```python
from build123d import *

# Parameters (mm, degrees)
F0_R     = 2.921
F1_DEPTH = 50.8
F3_DEPTH = 278.638
F4_R     = 5.08
F6_DEPTH = 79.502
F9_DEPTH = 68.072


with BuildPart() as f1:
    # F0 (on Front) → F1 (new body)
    with BuildSketch(Plane.XZ):
        Polygon((25.4, 69.85), (0, 0), (127, 0), (101.6, 69.85), align=None)
        with Locations((38.1, 53.975)):
            Circle(F0_R, mode=Mode.SUBTRACT)
        with Locations((88.9, 53.975)):
            Circle(F0_R, mode=Mode.SUBTRACT)
    extrude(amount=F1_DEPTH)

    # F2 (on Right) → F3 (cut)
    with BuildSketch(Plane.YZ):
        with BuildLine():
            Line((-38.354, 86.910382), (-38.354, 38.354))
            ThreePointArc((-38.354, 38.354), (-25.4, 25.4), (-12.446, 38.354))
            Line((-12.446, 38.354), (-12.446, 88.236041))
            Line((-12.446, 88.236041), (-38.354, 86.910382))
        make_face()
    extrude(amount=F3_DEPTH, mode=Mode.SUBTRACT)

    # F4
    f4_edges = [f1.edges().sort_by_distance(p)[0] for p in [
        (114.3, -50.8, 34.925),
        (63.5, -50.8, 69.85),
        (12.7, -50.8, 34.925),
        (101.6, -44.577, 69.85),
        (101.6, -6.223, 69.85),
        (25.4, -44.577, 69.85),
        (25.4, -6.223, 69.85),
        (63.5, 0, 69.85),
        (114.3, 0, 34.925),
        (12.7, 0, 34.925),
    ]]
    fillet(f4_edges, radius=F4_R)

    # F5 (on face) → F6 (cut)
    with BuildSketch(Plane(origin=(0, 0, 0), x_dir=(1, 0, 0), z_dir=(0, 0, -1))):
        with BuildLine():
            Line((28.321, 25.4), (31.75, 25.4))
            Line((31.75, 25.4), (35.179, 25.4))
            ThreePointArc((35.179, 25.4), (31.75, 28.829), (28.321, 25.4))
        make_face()
        with BuildLine():
            Line((35.179, 25.4), (31.75, 25.4))
            Line((31.75, 25.4), (28.321, 25.4))
            ThreePointArc((28.321, 25.4), (31.75, 21.971), (35.179, 25.4))
        make_face()
        with BuildLine():
            ThreePointArc((98.679, 25.4), (95.25, 28.829), (91.821, 25.4))
            ThreePointArc((91.821, 25.4), (95.25, 21.971), (98.679, 25.4))
        make_face()
    extrude(amount=-F6_DEPTH, mode=Mode.SUBTRACT)

    # F8 (on offset) → F9 (cut)
    with BuildSketch(Plane.XY.offset(12.7)):
        with BuildLine():
            ThreePointArc((40.64, -25.4), (31.75, -16.51), (22.86, -25.4))
            Line((22.86, -25.4), (31.75, -25.4))
            Line((31.75, -25.4), (40.64, -25.4))
        make_face()
        with BuildLine():
            ThreePointArc((104.14, -25.4), (95.25, -16.51), (86.36, -25.4))
            ThreePointArc((86.36, -25.4), (95.25, -34.29), (104.14, -25.4))
        make_face()
        with BuildLine():
            Line((31.75, -25.4), (22.86, -25.4))
            ThreePointArc((22.86, -25.4), (31.75, -34.29), (40.64, -25.4))
            Line((40.64, -25.4), (31.75, -25.4))
        make_face()
    extrude(amount=F9_DEPTH, mode=Mode.SUBTRACT)


solid = f1.part
```
Part model, mm, in its own coordinate system. A direction names the side the tool comes from. Round coordinates to 2 decimals unless told otherwise and drop trailing zeros. Loops run counter-clockwise (first coordinate to the right, second up) from the corner with the lowest first, then second, coordinate; pieces in that order, holes last.
1. Flat gauge pins, fed straight in: pin 1 (5.5 mm diameter, centred on x = 96.5, y = -25.5, fed in from +Z); pin 2 (7.5 mm diameter, centred on x = 38.1, z = 53.975, fed in from +Y); pin 3 (4.5 mm diameter, centred on x = 88.9, z = 53.975, fed in from -Y); pin 4 (4 mm diameter, centred on y = -41, z = 60, fed in from +X). Where does each tip first touch, or does it go through?
Solutions:
pin 1: stops at z = 12.7
pin 2: stops at y = 0
pin 3: passes through
pin 4: stops at x = 105.91
2. Slice it at A-A (y = -25.4). Give the cut face in (x, z).
Solutions:
outline: (0, 0) - (28.32, 0) - (28.32, 12.7) - (22.86, 12.7) - (22.86, 25.4) - (9.24, 25.4) - close; (35.18, 0) - (91.82, 0) - (91.82, 12.7) - (86.36, 12.7) - (86.36, 25.4) - (40.64, 25.4) - (40.64, 12.7) - (35.18, 12.7) - close; (98.68, 0) - (127, 0) - (117.76, 25.4) - (104.14, 25.4) - (104.14, 12.7) - (98.68, 12.7) - close
3. Drill centre lines: line 1 along Y through (x, z) = (45, 56); line 2 along Z through (x, y) = (38.1, -41.25); line 3 along X through (y, z) = (-25, 7). Where is each one in solid material? Low to high.
Solutions:
line 1: y = -50.8 to -38.35, -12.45 to 0
line 2: z = 0 to 51.05, 56.9 to 69.85
line 3: x = 2.55 to 28.34, 35.16 to 91.84, 98.66 to 124.45
4. Two-plate mould, pull along Z, no slides. Class faces 4 (the face through (38.805, -19.991, 20.702)), 5 (the face through (40.8, -44.49, 52.86)), 6 (the face through (117.764, -29.631, 25.398)): pulls with the +Z half, pulls with the -Z half, needs draft (parallel to the pull), parting line crosses it, or undercut.
Solutions:
face 4: needs draft
face 5: undercut
face 6: pulls with the +Z half
5. 3-axis set-ups, long thin cutter, end or side, ignore diameter. For faces 1 (the face through (32, -29, 12.7)), 2 (the face through (63, -12.446, 54)), 3 (the face through (93.668, -28.442, 6.261)): which of +Z, -Z, +X, -X, +Y, -Y reach the whole face in a straight line?
Solutions:
face 1: +Z
face 2: +Z, +X, -X
face 3: +Z, -Z
6. Slice it at C-C (x = 54.5). Give the cut face in (y, z), and give its area (3 significant figures).
Solutions:
outline: (-50.8, 0) - (0, 0) - (0, 64.77) arc R5.08 ccw to (-5.08, 69.85) - (-12.45, 69.85) - (-12.45, 38.35) arc R12.95 cw to (-38.35, 38.35) - (-38.35, 69.85) - (-45.72, 69.85) arc R5.08 ccw to (-50.8, 64.77) - close
area: 2,460 mm2
7. Slice it at D-D (y = -11). Give the cut face in (x, z) (3 decimals), and give its area (3 significant figures).
Solutions:
outline: (0, 0) - (127, 0) - (102.816, 66.506) arc R5.08 ccw to (98.042, 69.85) - (28.958, 69.85) arc R5.08 ccw to (24.184, 66.506) - close; hole circle Ø5.842 at (38.1, 53.975); hole circle Ø5.842 at (88.9, 53.975)
area: 7,040 mm2
8. Slice it at B-B (x = 95.25). Give the cut face in (y, z), and give its area (3 significant figures).
Solutions:
outline: (-50.8, 0) - (-28.83, 0) - (-28.83, 12.7) - (-34.29, 12.7) - (-34.29, 28.93) arc R12.95 cw to (-38.35, 38.35) - (-38.35, 69.85) - (-45.72, 69.85) arc R5.08 ccw to (-50.8, 64.77) - close; (-21.97, 0) - (0, 0) - (0, 64.77) arc R5.08 ccw to (-5.08, 69.85) - (-12.45, 69.85) - (-12.45, 38.35) arc R12.95 cw to (-16.51, 28.93) - (-16.51, 12.7) - (-21.97, 12.7) - close
area: 2,130 mm2
